Autodesk Inventor part; units mm, degrees
ref_plane "YZ Plane" through (0, 0, 0) normal (1, 0, 0) x (0, 1, 0)
ref_plane "XZ Plane" through (0, 0, 0) normal (0, 1, 0) x (-1, 0, 0)
ref_plane "XY Plane" through (0, 0, 0) normal (0, 0, 1) x (1, 0, 0)
sketch "Sketch1" plane through (0, 0, 0) normal (0, 0, 1) x (1, 0, 0)
  circle A0 centre (0, 0) radius 4.7625
  dimension "d0" = 9.525
extrude "Extrusion1" add sketch "Sketch1" along normal blind 1.6866
sketch "Sketch2" plane through (0, 0, 1.6866) normal (0, 0, 1) x (1, 0, 0)
  circle A0 centre (0, 0) radius 4.7625
  line L0 (-4.7625, 0) -> (-3.937, 0)
  circle A1 centre (0, 0) radius 3.937
  dimension "d3" = 0.8255
extrude "Extrusion2" add sketch "Sketch2" along normal blind 10.8687 contours A1
sketch "Sketch3" plane through (0, 0, 12.5552) normal (0, 0, 1) x (1, 0, 0)
  circle A0 centre (0, 0) radius 2.3368
  dimension "d6" = 4.6736
extrude "Extrusion3" cut sketch "Sketch3" against normal blind 31.9938
properties part number "Bushing" material "Copper, Cast"
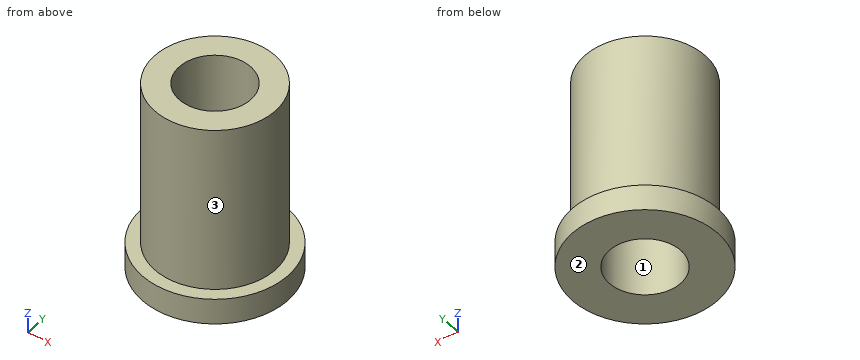
Geometry: final body of the model. Coordinates: model frame, mm. Face numbers are marked on the shaded views. Give positions to 0.01 mm unless a question says otherwise; leave off trailing zeros. Write each loop counter-clockwise with the first axis right and the second up, starting at its lowest first coordinate (ties: lowest second). Pieces come first, ordered by that corner, then holes.
(1) Mould query, pull axis Y, two halves, no side actions, for the marked faces 1, 2 and 3. Classes: released by +Y, released by -Y, zero draft, split by the parting line, or undercut.
(2) Cut plane D-D, the plane y = 3. Return loops of the section in (x, z).
(3) Cut plane B-B, the plane x = 0. Return loops of the section in (y, z).
(4) First-contact query: P1, Ø2, axis at y = 2, z = 11, coming from the -X side; P2, Ø5.5, axis at x = 0, y = 0, coming from the +Z side; P3, Ø1.5, axis at y = 3, z = 9, coming from the -X side; P4, Ø4, axis at y = 2.5, z = 7.5, coming from the -X side. Flat tips, straight axial feed; report the tip coordinate or a pass-through.
(5) Ray query, line 1 (Y direction, x = 0, z = 9); line 2 (Z direction, x = -4, y = 2.5); line 3 (Y direction, x = -1, z = 8). Return the intervals inside material, ascending.
(6) Cut plane A-A, the plane y = 1.5. Return loops of the section in (x, z), then the cut area to 3 significant figures.
(7) Cut plane C-C, the plane z = 4. Return loops of the section in (x, y).
Values follow:
1. face 1: undercut
1. face 2: zero draft
1. face 3: split by the parting line
2. outline: (-3.7, 0) - (3.7, 0) - (3.7, 1.69) - (2.55, 1.69) - (2.55, 12.56) - (-2.55, 12.56) - (-2.55, 1.69) - (-3.7, 1.69) - close
3. outline: (-4.76, 0) - (-2.34, 0) - (-2.34, 12.56) - (-3.94, 12.56) - (-3.94, 1.69) - (-4.76, 1.69) - close; (2.34, 0) - (4.76, 0) - (4.76, 1.69) - (3.94, 1.69) - (3.94, 12.56) - (2.34, 12.56) - close
4. P1: stops at x = -3.81
4. P2: stops at z = 12.56
4. P3: stops at x = -3.23
4. P4: stops at x = -3.91
5. line 1: y = -3.94 to -2.34, 2.34 to 3.94
5. line 2: z = 0 to 1.69
5. line 3: y = -3.81 to -2.11, 2.11 to 3.81
6. outline: (-4.52, 0) - (-1.79, 0) - (-1.79, 12.56) - (-3.64, 12.56) - (-3.64, 1.69) - (-4.52, 1.69) - close; (1.79, 0) - (4.52, 0) - (4.52, 1.69) - (3.64, 1.69) - (3.64, 12.56) - (1.79, 12.56) - close
6. area: 49.4 mm2
7. outline: circle Ø7.87 at (0, 0); hole circle Ø4.67 at (0, 0)
